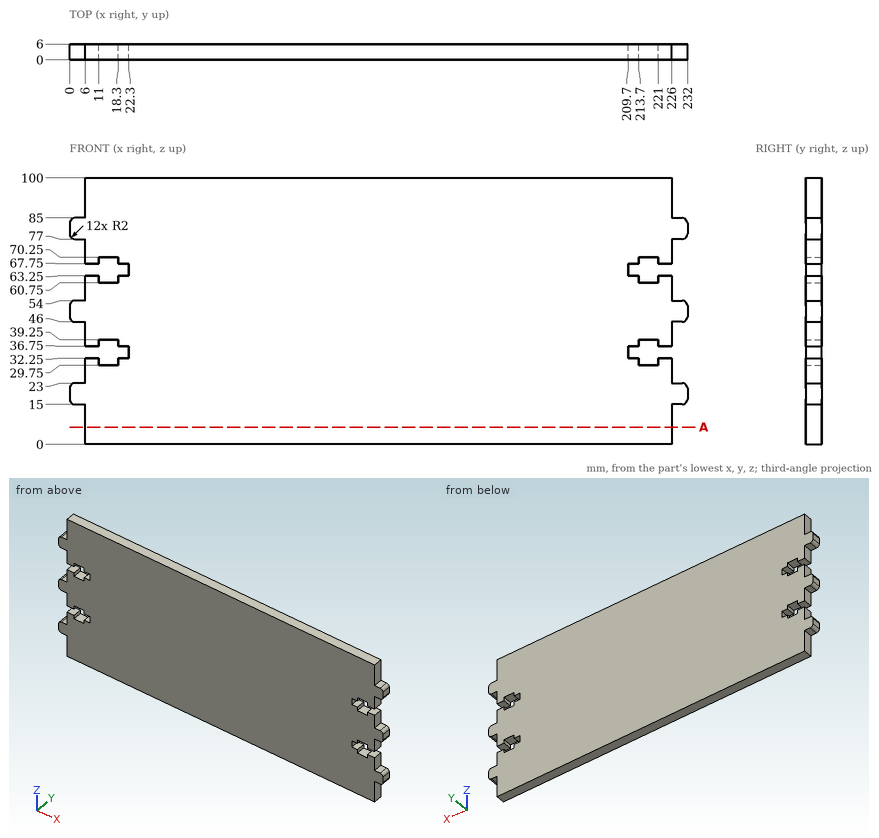
Study the drawing (mm; zero at the part's minimum x, y, z) and answer. Give positions to 0.01 mm unless a question says otherwise; leave off trailing zeros. Order: outer loops, then holes, each group sorted by start corner. A loop starts at its lowest first (then second) coordinate and runs counter-clockwise, first axis right, second up. Notation, with made-up numbers: (18, 63.5) -> (72, 63.5) arc R13 cw to (72, 84.5) -> close; hole circle Ø9 at (-39.5, 51). An arc over 180 degrees is marked (long way). Put each result on its own line as item: value.
Item 1: Straight lines are drawn through the part: line 1 (Z direction, x = 10, y = 3); line 2 (Z direction, x = 214, y = 1.2); line 3 (X direction, y = 5, z = 31.5). For each, find the intervals that lie inside material, in ascending order.
Established:
line 1: z = 0 to 32.25, 36.75 to 63.25, 67.75 to 100
line 2: z = 0 to 29.75, 39.25 to 60.75, 70.25 to 100
line 3: x = 6 to 11, 18.3 to 213.7, 221 to 226
Item 2: Given P1, Ø0.8, axis at y = 1.5, z = 31.5, coming from the -X side; P2, Ø1.8, axis at y = 4, z = 59.5, coming from the +X side, each flat-ended and moving along its own axis, determine where each tip first touches the part or whether it passes through.
Established:
P1: stops at x = 6
P2: stops at x = 226
Item 3: A cutting plane is placed at A-A on z = 6.5. Give the vertices of the cut face in (x, y), plus the area to 3 significant figures.
Established:
outline: (6, 0) -> (226, 0) -> (226, 6) -> (6, 6) -> close
area: 1,320 mm^2
